Build history of the part. All positions in model axes, mm. Face numbers are marked on the shaded views. A direction names the side the tool comes from. Coordinates: 2 decimals unless noted, no trailing zeros. Loops run counter-clockwise (first coordinate to the right, second up) from the corner with the lowest first, then second, coordinate; pieces in that order, holes last.
(1) Flat gauge pins, fed straight in: P1, Ø2.5, axis at x = 606, y = 2.5, coming from the -Z side; P2, Ø1.5, axis at y = 137, z = -123.5, coming from the -X side. Where does each tip first touch, or does it go through?
(2) Slice it at A-A (z = -257.5). Give the cut face in (x, y), and give its area (3 significant figures).
(3) Slice it at D-D (x = 531.5). Give the cut face in (y, z), and give its area (3 significant figures).
(4) Tool access for the marked faces 1 and 2: list every direction of +Z, -Z, +X, -X, +Y, -Y with a clear straight run to the whole face (end or side of a thin tool).
(5) Slice it at C-C (y = 184.5). Give the cut face in (x, z), and give its area (3 significant figures).
(6) Wall check: L1, parallel to X at y = 209.5, z = -506; L2, parallel to Y at x = 1247.5, z = -479; L3, parallel to X at y = 53.5, z = -51. Give the ranges that are in metal, low to high.
(7) Slice it at B-B (z = -118). Give the cut face in (x, y).
from build123d import *

# Parameters (mm, degrees)
F1_DEPTH = 600
F3_DEPTH = 5


with BuildPart() as f1:
    # F0 (on Top) → F1 (new body)
    with BuildSketch(Plane.XY):
        with BuildLine():
            Line((0, 5), (0, 0))
            Line((0, 0), (1400, 0))
            ThreePointArc((1400, 0), (1509.601551, 45.398449), (1555, 155))
            Line((1555, 155), (1555, 320))
            Line((1555, 320), (1550, 320))
            Line((1550, 320), (1550, 155))
            ThreePointArc((1550, 155), (1506.066017, 48.933983), (1400, 5))
            Line((1400, 5), (0, 5))
        make_face()
    extrude(amount=-F1_DEPTH)

    # F2 (on face) → F3 (cut)
    with BuildSketch(Plane.XZ):
        with BuildLine():
            Line((320, -312.450663), (193.687297, -571.887334))
            ThreePointArc((193.687297, -571.887334), (175.243069, -592.393199), (148.73238, -600))
            Line((148.73238, -600), (1128.666073, -600))
            ThreePointArc((1128.666073, -600), (1099.524718, -590.62981), (1081.305765, -566.031258))
            Line((1081.305765, -566.031258), (991.900594, -301.906227))
            ThreePointArc((991.900594, -301.906227), (937.243734, -228.110571), (849.81967, -200))
            Line((849.81967, -200), (499.81967, -200))
            ThreePointArc((499.81967, -200), (393.776913, -230.427202), (320, -312.450663))
        make_face()
    extrude(amount=-F3_DEPTH, mode=Mode.SUBTRACT)


solid = f1.part
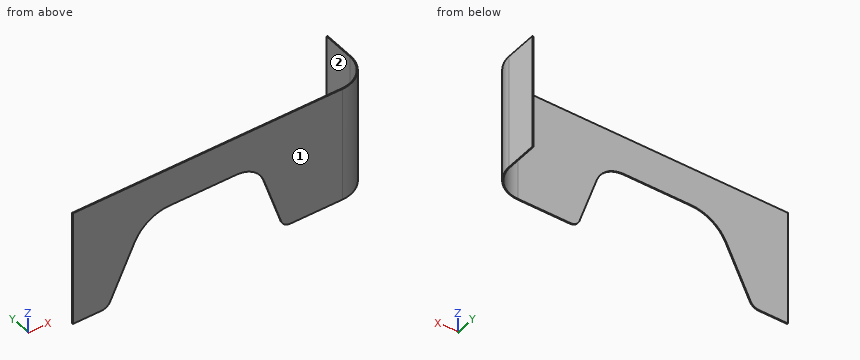
Response values:
1. P1: stops at z = -200
1. P2: stops at x = 1548.82
2. outline: (0, 0) - (359.49, 0) - (359.49, 5) - (0, 5) - close; (967.9, 0) - (1400, 0) arc R155 ccw to (1555, 155) - (1555, 320) - (1550, 320) - (1550, 155) arc R150 cw to (1400, 5) - (967.9, 5) - close
2. area: 5,980 mm2
3. outline: (0, -200) - (5, -200) - (5, 0) - (0, 0) - close
3. area: 1,000 mm2
4. face 1: +Z, -Z, +X, -X, -Y
4. face 2: +Z, -Z, -X, +Y
5. outline: (1550, -600) - (1555, -600) - (1555, 0) - (1550, 0) - close
5. area: 3,000 mm2
6. L1: x = 1550 to 1555
6. L2: y = 0 to 5
6. L3: x = 1510.44 to 1517.14
7. outline: (0, 0) - (1400, 0) arc R155 ccw to (1555, 155) - (1555, 320) - (1550, 320) - (1550, 155) arc R150 cw to (1400, 5) - (0, 5) - close
